Check sheet for the modelled part. Datum: model origin and axes. Units: mm. Give positions to 0.01 mm unless a question says otherwise; leave off trailing zeros. Loops run counter-clockwise (first coordinate to the right, second up) from the corner with the lowest first, then second, coordinate; pieces in that order, holes last. Notation, with made-up numbers: (-32.5, 71.5) - (-7.5, 71.5) arc R16 ccw to (-7.5, 94.5) - close; hole circle Ø4 at (-27, 28). An arc over 180 degrees is marked (long way). Answer in a Markdown table with one row per item. Add a question column.
(1) Sectioned sample at A-A on z = 2.25. State how many separate pieces and enclosed holes the cut face has, then the cut area to 3 significant figures.
(2) Draft check along X on faces 1 (the face through (230.306, 92.362, 1.521)), 2 (the face through (227, 59, 0)), 3 (the face through (371.26, 111.975, 1.479)). Enter one of: released by +X, released by -X, zero draft, split by the parting line, or undercut.
(3) Thickness scan on L1, parallel to Y at x = 193, z = 2; L2, parallel to Y at x = 201, z = 0.9; L3, parallel to Y at x = 333.5, z = 1.4. Record the ranges inside material, lowest first.
(4) Go/stop test with flat-tipped pins: P1, Ø1.5, axis at y = 120, z = 2, coming from the -X side; P2, Ø2.5, axis at x = 119, y = 55, coming from the +Z side; P3, Ø0.9, axis at y = 135, z = 1.5, coming from the +X side. Record where each tip stops, or that it passes through.
(5) Sectioned sample at C-C on x = 63. Enter the section's corners in (y, z).
(6) Sectioned sample at B-B on y = 80. Enter the section's corners in (x, z).
from build123d import *

# Parameters (mm, degrees)
Y_KSEKLIK_EKSTR_ZYON1_DEPTH = 3
IZIM2_R                     = 2
KES_EKSTR_ZYON1_DEPTH       = 3


with BuildPart() as part:
    # Çizim1 → Yükseklik-Ekstrüzyon1 (new body)
    with BuildSketch(Plane.XY):
        Polygon((0, 0), (460, 0), (460, 75), (280, 150), (180, 150), (0, 75), align=None)
    extrude(amount=Y_KSEKLIK_EKSTR_ZYON1_DEPTH)

    # Çizim2 → Kes-Ekstrüzyon1 (cut)
    with BuildSketch(Plane.XY.offset(3)):
        with Locations((45, 55)):
            Circle(IZIM2_R)
        with Locations((119, 55)):
            Circle(IZIM2_R)
        with Locations((193, 55)):
            Circle(IZIM2_R)
        with Locations((267, 55)):
            Circle(IZIM2_R)
        with Locations((341, 55)):
            Circle(IZIM2_R)
        with Locations((415, 55)):
            Circle(IZIM2_R)
        with Locations((201, 130)):
            Circle(IZIM2_R)
        with Locations((259, 130)):
            Circle(IZIM2_R)
        with BuildLine():
            Line((210, 150), (250, 150))
            Line((250, 150), (250, 100))
            ThreePointArc((250, 100), (230, 92.360679775), (210, 100))
            Line((210, 100), (210, 150))
        make_face()
    extrude(amount=-KES_EKSTR_ZYON1_DEPTH, mode=Mode.SUBTRACT)


solid = part.part
Reply:
| question | item | result |
|---|---|---|
| 1 | separate pieces | 1 |
| 1 | enclosed holes | 8 |
| 1 | area | 53,200 mm^2 |
| 2 | face 1 | undercut |
| 2 | face 2 | zero draft |
| 2 | face 3 | released by +X |
| 3 | L1 | 0 to 53, 57 to 150 |
| 3 | L2 | 0 to 128, 132 to 150 |
| 3 | L3 | 0 to 127.71 |
| 4 | P1 | x = 106.2 |
| 4 | P2 | through |
| 4 | P3 | x = 317.08 |
| 5 | outline | (0, 0) - (101.25, 0) - (101.25, 3) - (0, 3) - close |
| 6 | outline | (12, 0) - (448, 0) - (448, 3) - (12, 3) - close |
